The listing builds one solid part. Answer for the finished solid, in the listing's coordinates (mm). A direction names the side the tool comes from. Round coordinates to 2 decimals unless told otherwise and drop trailing zeros. Order: outer loops, then holes, each group sorted by start corner. A loop starts at its lowest first (then second) coordinate and runs counter-clockwise, first axis right, second up. Notation, with made-up numbers: (3.25, -24.75) -> (7.25, -24.75) arc R13 cw to (7.25, -2.75) -> close; hole circle Ø10 at (-13, 75.25). An arc over 180 degrees is marked (long way). Return JSON: item names as keys, results as strings. Group by question number.
(1) Which of the six approach directions +Z, -Z, +X, -X, +Y, -Y give full straight-line access (tool end or side, diameter ignored) to faces 1 (the face through (-4.686, 35.694, 0.493)), 2 (the face through (-1, 1, 150))?
(2) Each of these flat-tipped pins is pushed along its axis until it touches: pin 1 (5 mm diameter, centred on x = -27, z = 33, fed in from -Y); pin 2 (10 mm diameter, centred on x = 12, z = 130, fed in from -Y); pin 3 (4 mm diameter, centred on x = -10.5, z = 96.5, fed in from -Y). Where does it stop, or does it pass through?
(3) The part is cut by section C-C (z = 12). Determine the outline of the cut face in (x, y).
(4) The part is cut by section A-A (x = 14.5). Determine the outline of the cut face in (y, z).
(5) The part is cut by section B-B (y = -18.5). Determine the outline of the cut face in (x, z), plus the area to 3 significant figures.
(6) Determine the mould class of faces 3 (the face through (-30, 19, 1)), 4 (the face through (47.69, 15.02, 73.95)), 5 (the face through (22, -33, 0)) for opening direction X: +X half, -X half, draft (parallel to the pull), parting line (faces both ways), or undercut.
(7) Consider line 1 (Y direction, x = 0, z = 0.8); line 2 (Y direction, x = -2, z = 126.5); line 3 (Y direction, x = -8, z = 23). Determine where each line is inside the solid, lowest interval first. Write a range as [from, to].
from build123d import *

# Parameters (mm, degrees)
F2_R     = 50
F3_DEPTH = 150
F4_R     = 36
F4_R_2   = 35
F5_DEPTH = 1


with BuildPart() as f3:
    # F2 (on Top) → F3 (new body)
    with BuildSketch(Plane.XY):
        Circle(F2_R)
    extrude(amount=F3_DEPTH)

    # F4 (on Top) → F5 (cut)
    with BuildSketch(Plane.XY):
        Circle(F4_R)
        Circle(F4_R_2, mode=Mode.SUBTRACT)
    extrude(amount=F5_DEPTH, mode=Mode.SUBTRACT)


solid = f3.part
Answer below:
{
 "1": {"face 1": "-Z", "face 2": "+Z, +X, -X, +Y, -Y"},
 "2": {"pin 1": "stops at y = -43.59", "pin 2": "stops at y = -49.51", "pin 3": "stops at y = -49.27"},
 "3": {"outline": "circle Ø100 at (0, 0)"},
 "4": {"outline": "(-47.85, 0) -> (-32.95, 0) -> (-32.95, 1) -> (-31.86, 1) -> (-31.86, 0) -> (31.86, 0) -> (31.86, 1) -> (32.95, 1) -> (32.95, 0) -> (47.85, 0) -> (47.85, 150) -> (-47.85, 150) -> close"},
 "5": {"outline": "(-46.45, 0) -> (-30.88, 0) -> (-30.88, 1) -> (-29.71, 1) -> (-29.71, 0) -> (29.71, 0) -> (29.71, 1) -> (30.88, 1) -> (30.88, 0) -> (46.45, 0) -> (46.45, 150) -> (-46.45, 150) -> close", "area": "13,900 mm²"},
 "6": {"face 3": "undercut", "face 4": "parting line", "face 5": "draft"},
 "7": {"line 1": "y = [-50, -36], [-35, 35], [36, 50]", "line 2": "y = [-49.96, 49.96]", "line 3": "y = [-49.36, 49.36]"}
}
